Geometry: final body of the model. Coordinates: model frame, mm. A direction names the side the tool comes from. Coordinates: 2 decimals unless noted, no trailing zeros. Write each loop counter-clockwise with the first axis right and the second up, starting at its lowest first coordinate (ties: lowest second). Pieces come first, ordered by that corner, then holes. Notation, with made-up numbers: (-10, 31) - (45, 31) arc R18 cw to (45, 54) - close; hole circle Ø10 at (11, 74). An arc over 180 degrees is marked (long way). Put each result on its own line as item: value.
```python
from build123d import *

# Parameters (mm, degrees)
F1_DEPTH  = 7
F2_W      = 4
F2_H      = 12
F3_DEPTH  = 8
F4_W      = 12.2146774828
F4_H      = 1.6385169476
F5_DEPTH  = 8
F7_DEPTH  = 80
F8_R      = 2.25
F9_DEPTH  = 25
F10_W     = 40
F10_H     = 30
F10_R     = 2.25
F11_DEPTH = 4
F12_R     = 3


with BuildPart() as f1:
    # F0 (on Top) → F1 (new body)
    with BuildSketch(Plane.XY):
        Polygon((-29, 15), (-33, 15), (-33, -1), (-45, -1), (-45, -15), (45, -15), (45, 15), (29, 15), align=None)
        with BuildLine():
            ThreePointArc((-28.25, 10), (-29.5303300859, 9.4696699141), (-29, 10.75))
            ThreePointArc((-29, 10.75), (-28.4696699141, 10.5303300859), (-28.25, 10))
        make_face(mode=Mode.SUBTRACT)
        with BuildLine():
            ThreePointArc((29.75, 10), (28.4696699141, 9.4696699141), (29, 10.75))
            ThreePointArc((29, 10.75), (29.5303300859, 10.5303300859), (29.75, 10))
        make_face(mode=Mode.SUBTRACT)
    extrude(amount=F1_DEPTH)

    # F2 (on face) → F3 (join)
    with BuildSketch(Plane.XY.offset(7)):
        Polygon((-33, -1), (-45, -1), (-45, -15), (-32.7853225172, -15), (-32.7853225172, -1), align=None)
        with Locations((43, -9)):
            Rectangle(F2_W, F2_H)
    extrude(amount=F3_DEPTH)

    # F4 (on face) → F5 (cut)
    with BuildSketch(Plane.XY.offset(15)):
        with Locations((-38.8926612586, -1.8192584738)):
            Rectangle(F4_W, F4_H)
    extrude(amount=-F5_DEPTH, mode=Mode.SUBTRACT)

    # F6 (on face) → F7 (cut)
    with BuildSketch(Plane.YZ.offset(45)):
        with BuildLine():
            ThreePointArc((-12.5, 9.4), (-11.3686291501, 9.8686291501), (-10.9, 11))
            ThreePointArc((-10.9, 11), (-13.6313708499, 12.1313708499), (-12.5, 9.4))
        make_face()
    extrude(amount=-F7_DEPTH, mode=Mode.SUBTRACT)

    # F8 (on face) → F9 (cut)
    with BuildSketch(Plane.XY.offset(7)):
        with Locations((-10, 0)):
            Circle(F8_R)
        with BuildLine():
            ThreePointArc((12.25, 0), (10, 2.25), (7.75, 0))
            ThreePointArc((7.75, 0), (10, -2.25), (12.25, 0))
        make_face()
    extrude(amount=-F9_DEPTH, mode=Mode.SUBTRACT)

    # F10 (on face) → F11 (cut)
    with BuildSketch(Plane.XY.offset(7)):
        Rectangle(F10_W, F10_H)
        with Locations((-10, 0)):
            Circle(F10_R, mode=Mode.SUBTRACT)
        with Locations((10, 0)):
            Circle(F10_R, mode=Mode.SUBTRACT)
    extrude(amount=-F11_DEPTH, mode=Mode.SUBTRACT)

    # F12
    f12_edges = [f1.edges().sort_by_distance(p)[0] for p in [
        (-38.892661, -15, 15),
        (43, -15, 15),
        (-38.892661, -2.638517, 15),
        (43, -3, 15),
    ]]
    fillet(f12_edges, radius=F12_R)


solid = f1.part
```
1. Ray query, probe 1 along X at (y, z) = (-9, 14); probe 2 along Y at (x, z) = (42.15, 11); probe 3 along X at (y, z) = (10, 4.25). Return the intervals inside material, ascending. Write a range as from..to.
Answer below:
probe 1: x = -45..-32.79, 41..45
probe 2: y = -15..-14.1, -10.9..-3
probe 3: x = -33..-29.75, -28.25..-20, 20..28.25, 29.75..45
2. Section query B-B (x = -10). Return loops of the section in (y, z).
Answer below:
outline: (-15, 0) - (-2.25, 0) - (-2.25, 3) - (-15, 3) - close; (2.25, 0) - (15, 0) - (15, 3) - (2.25, 3) - close
3. Set-up query: faces 1 (the flat face through (-39, -9, 15)), 2 (the flat face through (-39, -2.639, 10)), 3 (the flat face through (-32.785, -9, 11)), 4 (the cylindrical face through (43.03, -3.9, 14.14)), 5 (the flat face through (-33, 7, 3)). Return all of +Z, -Z, +X, -X, +Y, -Y with unobstructed straight access to the full face (end or side cutting, diameter ignored); none if empty.
Answer below:
face 1: +Z, +X, -X, +Y, -Y
face 2: +Z, +X, -X, +Y
face 3: +Z, +Y, -Y
face 4: +Z, +X, +Y
face 5: +Z, -Z, -X, +Y
4. Pin query (flat end, axial travel): pin 1 Ø5.5 at (x, z) = (-41, 4) entering from +Y; pin 2 Ø10 at (x, y) = (-8.5, -5) entering from -Z; pin 3 Ø2.5 at (y, z) = (-12.5, 11) entering from +X; pin 4 Ø2 at (y, z) = (5, 2.5) entering from -X. Return the tip coordinate at first contact, or that it passes through.
Answer below:
pin 1: stops at y = -1
pin 2: stops at z = 0
pin 3: stops at x = -35
pin 4: stops at x = -33
5. Section query C-C (x = 26). Return loops of the section in (y, z).
Answer below:
outline: (-15, 0) - (15, 0) - (15, 7) - (-15, 7) - close
6. Section query A-A (y = 0). Return loops of the section in (x, z).
Answer below:
outline: (-33, 0) - (-12.25, 0) - (-12.25, 3) - (-20, 3) - (-20, 7) - (-33, 7) - close; (-7.75, 0) - (7.75, 0) - (7.75, 3) - (-7.75, 3) - close; (12.25, 0) - (45, 0) - (45, 7) - (20, 7) - (20, 3) - (12.25, 3) - close
7. Mould query, pull axis Z, two halves, no side actions, for faces 6 (the flat face through (-1, 0, 0)), 7 (the flat face through (-35, -13, 11)), 8 (the flat face through (43, -9, 15)), 9 (the flat face through (20, 0, 5)). Classes: +Z half, -Z half, draft (parallel to the pull), parting line (faces both ways), or undercut.
Answer below:
face 6: -Z half
face 7: undercut
face 8: +Z half
face 9: draft
